Build history of the part. All positions in model axes, mm. A direction names the side the tool comes from. Round coordinates to 2 decimals unless told otherwise and drop trailing zeros. Write each loop counter-clockwise with the first axis right and the second up, starting at its lowest first coordinate (ties: lowest second). Pieces come first, ordered by that corner, then holes. Notation, with made-up numbers: (35, 36) - (61, 36) arc R22 cw to (61, 42) - close; hole circle Ø2 at (-1, 23.5). An arc over 180 degrees is marked (long way). One line per question, with ' | ' between items.
from build123d import *

# Parameters (mm, degrees)
SKETCH1_R     = 5
CORPO_DEPTH   = 90
ABA_START     = -7
ABA_1MM_DEPTH = 7


with BuildPart() as part:
    # Sketch1 → Corpo (new body)
    with BuildSketch(Plane(origin=(0, 0, 0), x_dir=(0, 0, -1), z_dir=(1, 0, 0))):
        with Locations(Location((0, 0, 0), (0, 0, 180))):
            Circle(SKETCH1_R)
    extrude(amount=CORPO_DEPTH)

    # Sketch2 → Aba 1mm (cut)
    with BuildSketch(Plane(origin=(90, 0, 0), x_dir=(0, 0, -1), z_dir=(1, 0, 0)).offset(ABA_START)):
        with BuildLine():
            ThreePointArc((-0.5, 4.974937186), (-5, 0), (-0.5, -4.974937186))
            Line((-0.5, -4.974937186), (-0.5, 4.974937186))
        make_face()
        with BuildLine():
            Line((0.5, 4.974937186), (0.5, -4.974937186))
            ThreePointArc((0.5, -4.974937186), (3.708099244, -3.354101966), (5, 0))
            ThreePointArc((5, 0), (3.708099244, 3.354101966), (0.5, 4.974937186))
        make_face()
    extrude(amount=ABA_1MM_DEPTH, mode=Mode.SUBTRACT)


solid = part.part
Q1. Drill centre lines: L1, parallel to X at y = 0.75, z = -0.75; L2, parallel to Z at x = 85, y = 1.5; L3, parallel to Y at x = 16, z = -0.5. Where is each one in solid material? Low to high. Write a range as from..to.
Found:
L1: 0..83 | L2: -0.5..0.5 | L3: -4.97..4.97
Q2. Which spindle directions (+Z, -Z, +X, -X, +Y, -Y) get a long thin tool onto all of the face, cutting with end or side? Do faces 1 (the flat face through (0, 0, 0)), 2 (the flat face through (86, 0, -0.5)), 3 (the flat face through (83, 0, 2)). Say none if no direction does.
Found:
face 1: +Z, -Z, -X, +Y, -Y | face 2: -Z, +X, +Y, -Y | face 3: +Z, +X, +Y, -Y
Q3. Saw through at D-D, the plane z = -3.75. List the corners of the cut face in (x, y).
Found:
outline: (0, -3.31) - (83, -3.31) - (83, 3.31) - (0, 3.31) - close
Q4. Saw through at B-B, the plane x = 61. List the corners of the cut face in (y, z).
Found:
outline: circle Ø10 at (0, 0)
Q5. Saw through at A-A, the plane y = 0. List the corners of the cut face in (x, z), then the cut area to 3 significant figures.
Found:
outline: (0, -5) - (83, -5) - (83, -0.5) - (90, -0.5) - (90, 0.5) - (83, 0.5) - (83, 5) - (0, 5) - close | area: 837 mm^2
Q6. Drop flat-ended pins along their axis: pin 1 (2 mm diameter, centred on x = 86, y = -2, fed in from +Z); pin 2 (6 mm diameter, centred on x = 10, z = 2, fed in from +Y); pin 3 (1.5 mm diameter, centred on x = 56, z = -3, fed in from +Y); pin 4 (3.5 mm diameter, centred on y = 0.5, z = 2.5, fed in from +X). Give the stop position or say it passes through.
Found:
pin 1: z = 0.5 | pin 2: y = 5 | pin 3: y = 4.47 | pin 4: x = 83
Q7. Saw through at C-C, the plane z = 4. List the corners of the cut face in (x, y).
Found:
outline: (0, -3) - (83, -3) - (83, 3) - (0, 3) - close
